from build123d import *

# Parameters (mm, degrees)
SALIENTE_EXTRUIR1_DEPTH           = 3
CROQUIS2_W                        = 120
CROQUIS2_H                        = 3
SALIENTE_EXTRUIR2_DEPTH           = 27
DI_METRO_DE_TALADRO_7_0_7_1_D     = 7
DI_METRO_DE_TALADRO_7_0_7_1_DEPTH = 30


with BuildPart() as part:
    # Croquis1 → Saliente-Extruir1 (new body)
    with BuildSketch(Plane.XY.offset(-77.120136034)):
        Polygon((-60, 662.649987793), (-60, 647.649987793), (60, 647.649987793), (60, 662.649987793), (45, 677.649987793), (-45, 677.649987793), align=None)
    extrude(amount=-SALIENTE_EXTRUIR1_DEPTH)

    # Croquis2 → Saliente-Extruir2 (add)
    with BuildSketch(Plane.XY.offset(-77.120136034)):
        with Locations((0, 649.149987793)):
            Rectangle(CROQUIS2_W, CROQUIS2_H)
    extrude(amount=SALIENTE_EXTRUIR2_DEPTH)

    # Diámetro de taladro Ø7.0 (7)1
    with Locations(Plane(origin=(0, 0, -80.120136034), x_dir=(-1, 0, 0), z_dir=(0, 0, -1))):
        with Locations((45, 664.649987793), (-45, 664.649987793)):
            Hole(DI_METRO_DE_TALADRO_7_0_7_1_D / 2, depth=DI_METRO_DE_TALADRO_7_0_7_1_DEPTH)


solid = part.part
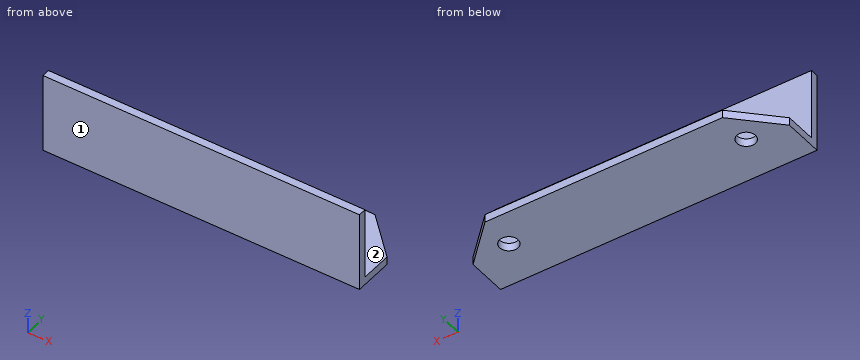
Work out the finished part from the listing and answer in its coordinate system (mm). Face numbers are marked on the shaded views. A direction names the side the tool comes from. Give positions to 0.01 mm unless a question says otherwise; leave off trailing zeros. Order: outer loops, then holes, each group sorted by start corner. A loop starts at its lowest first (then second) coordinate and runs counter-clockwise, first axis right, second up. Notation, with made-up numbers: (52, -13) -> (95, -13) arc R18 ccw to (95, 18) -> close; hole circle Ø11 at (-31.5, 20). An arc over 180 degrees is marked (long way). One line per item, written item: value.
Item 1: A tool of negligible diameter and unlimited length cuts with its end or side. For the marked faces 1 and 2, from which of +Z, -Z, +X, -X, +Y, -Y can it reach the whole face along a straight path? Write none if from no direction.
Answer sheet:
face 1: +Z, -Z, +X, -X, -Y
face 2: +Z, +X, -X, +Y
Item 2: Straight lines are drawn through the part: probe 1 along Y at (x, z) = (45, -78.1); probe 2 along Z at (x, y) = (-45, 670); probe 3 along Y at (x, z) = (54.5, -70.75). For each, find the intervals that lie inside material, in ascending order.
Answer sheet:
probe 1: 647.65 to 661.15, 668.15 to 677.65
probe 2: -80.12 to -77.12
probe 3: 647.65 to 650.65
Item 3: Flat-ended cylindrical pins translate along their axes: P1, Ø5, axis at x = 48, y = 667, coming from the +Z side; P2, Ø4, axis at x = 45, y = 664.65, coming from the -Z side (3 decimals); P3, Ø3, axis at x = -26.5, z = -56.5, coming from the +Y side; P4, Ø10, axis at x = 8.5, y = 652.5, coming from the +Z side. Find the tip coordinate at first contact, or state that the pin passes through.
Answer sheet:
P1: z = -77.12
P2: through
P3: y = 650.65
P4: z = -50.12
Item 4: Find section A-A, the plane x = -13.5. Give the vertices of the cut face in (y, z).
Answer sheet:
outline: (647.65, -80.12) -> (677.65, -80.12) -> (677.65, -77.12) -> (650.65, -77.12) -> (650.65, -50.12) -> (647.65, -50.12) -> close
Item 5: Find section B-B, the plane y = 654.25. Give the vertices of the cut face in (x, z).
Answer sheet:
outline: (-60, -80.12) -> (60, -80.12) -> (60, -77.12) -> (-60, -77.12) -> close
Item 6: Find section C-C, the plane z = -63. Give the vertices of the cut face in (x, y).
Answer sheet:
outline: (-60, 647.65) -> (60, 647.65) -> (60, 650.65) -> (-60, 650.65) -> close
